Geometry check sheet. Reference: the model listing, model coordinates, mm. A direction names the side the tool comes from. Coordinates: 2 decimals unless noted, no trailing zeros. Write each loop counter-clockwise with the first axis right and the second up, starting at its lowest first coordinate (ties: lowest second). Pieces come first, ordered by that corner, then holes. Notation, with made-up numbers: (10, 63) -> (31, 63) arc R8 cw to (31, 76) -> close; hole circle Ø4 at (34.5, 80). An arc over 180 degrees is marked (long way). Use a Markdown table: item, result.
```python
from build123d import *

# Parameters (mm, degrees)
BOSS_EXTRUDE1_REACH     = 19.38
SKETCH3_W               = 4.76
SKETCH3_H               = 0.63
CUT_EXTRUDE1_DEPTH      = 19.196319901
CUT_EXTRUDE1_DEPTH_BACK = 19.196319901
SKETCH4_R               = 0.5


with BuildPart() as part:
    # Sweep1: sweep along a path in Sketch2
    with BuildLine(Plane(origin=(0, 0, 0), x_dir=(1, 0, 0), z_dir=(0, 1, 0))) as sweep1_path:
        Line((0, 2.62), (7, 2.62))
        Line((7, 2.62), (11.415258217, 3.755932179))
        ThreePointArc((11.415258217, 3.755932179), (13.415796262, 6.491493797), (11.121440392, 8.985763424))
        Line((11.121440392, 8.985763424), (6.606732095, 9.62))
        Line((6.606732095, 9.62), (0, 9.62))
        Line((0, 9.62), (0, 2.62))
    # Sketch1 → Sweep1 (sweep)
    with BuildSketch(Plane(origin=(0, 0, 0), x_dir=(0, 0, -1), z_dir=(1, 0, 0))):
        with BuildLine():
            Line((2.62, 0), (3.74, 0))
            Line((3.74, 0), (3.74, 0.63))
            Line((3.74, 0.63), (3.167964646, 0.63))
            ThreePointArc((3.167964646, 0.63), (2.881836518, 1.458738594), (2.383379953, 2.18))
            Line((2.383379953, 2.18), (1.496179773, 2.18))
            ThreePointArc((1.496179773, 2.18), (1.478667505, 2.178597055), (1.46160194, 2.174424008))
            ThreePointArc((1.46160194, 2.174424008), (2.312336165, 1.231869091), (2.62, 0))
        make_face()
    sweep(path=sweep1_path.line, transition=Transition.RIGHT)

    # Sketch3 → Boss-Extrude1 (add, up to next)
    with BuildSketch(Plane(origin=(1.12, 0, 0), x_dir=(0, 0, -1), z_dir=(1, 0, 0)), mode=Mode.PRIVATE) as boss_extrude1_sk1:
        with Locations((6.12, 0.315)):
            Rectangle(SKETCH3_W, SKETCH3_H)
    boss_extrude1_tool1 = extrude(boss_extrude1_sk1.sketch, amount=BOSS_EXTRUDE1_REACH, mode=Mode.PRIVATE) - part.part
    add(boss_extrude1_tool1.solids().sort_by_distance((1.12, 0.315, -6.12))[0])

    # Sketch4 → Cut-Extrude1 (cut, two sides: drawn at the far end of the back side and taken through both)
    with BuildSketch(Plane(origin=(0, 0.63, 0), x_dir=(1, 0, 0), z_dir=(0, 1, 0)).offset(-CUT_EXTRUDE1_DEPTH_BACK)):
        with Locations(Location((10.75, 6.341726352, 0), (0, 0, 270))):
            Circle(SKETCH4_R)
        with BuildLine():
            Line((1.497140147, 7.12), (1.497140147, 5.12))
            ThreePointArc((1.497140147, 5.12), (2.204246928, 4.827106781), (2.497140147, 4.12))
            Line((2.497140147, 4.12), (4.497140147, 4.12))
            ThreePointArc((4.497140147, 4.12), (4.790033365, 4.827106781), (5.497140147, 5.12))
            Line((5.497140147, 5.12), (5.497140147, 7.12))
            ThreePointArc((5.497140147, 7.12), (4.790033365, 7.412893219), (4.497140147, 8.12))
            Line((4.497140147, 8.12), (2.497140147, 8.12))
            ThreePointArc((2.497140147, 8.12), (2.204246928, 7.412893219), (1.497140147, 7.12))
        make_face()
    extrude(amount=CUT_EXTRUDE1_DEPTH + CUT_EXTRUDE1_DEPTH_BACK, mode=Mode.SUBTRACT)


solid = part.part
```
Item 1: Section check C-C on z = -6. Count the separate pieces of the cut face and the enclosed holes in it, then the cut area to 3 significant figures.
Answer block:
| item | result |
|---|---|
| separate pieces | 3 |
| enclosed holes | 0 |
| area | 7.74 mm^2 |
Item 2: Mould release check, pull along X, two halves, no side actions. Record for faces 1 (the cylindrical face through (2.21, 0.31, -7.42)), 2 (the cylindrical face through (9.243, 1.216, -2.888)), 3 (the cylindrical face through (3.05, 1.22, -2.32)): +X half, -X half, draft (parallel to the pull), parting line (faces both ways), or undercut.
Answer block:
| item | result |
|---|---|
| face 1 | undercut |
| face 2 | +X half |
| face 3 | draft |
Item 3: Section check B-B on y = 0.8. Record the boundary of the cut face in (x, z).
Answer block:
| item | result |
|---|---|
| outline | (-0.13, -9.75) -> (6.62, -9.75) -> (11.14, -9.11) arc R2.8 ccw to (11.45, -3.63) -> (7.02, -2.49) -> (-0.13, -2.49) -> close; hole (0.51, -9.11) -> (6.57, -9.11) -> (11.05, -8.48) arc R2.16 ccw to (11.29, -4.25) -> (6.94, -3.13) -> (0.51, -3.13) -> close |
Item 4: Depth check by flat-ended pin: P1, Ø0.7, axis at y = 0.5, z = -6.5, coming from the -X side; P2, Ø0.5, axis at x = 4, y = 0, coming from the -Z side; P3, Ø3, axis at x = 6, z = -7, coming from the +Y side. Enter the tip coordinate at first touch or a pass-through.
Answer block:
| item | result |
|---|---|
| P1 | stops at x = -0.14 |
| P2 | stops at z = -9.63 |
| P3 | stops at y = 0.63 |
Item 5: Thickness scan on L1, parallel to Y at x = 2, z = -3.75; L2, parallel to X at y = 2, z = -5.5; L3, parallel to Z at x = 10.75, y = 0.2. Record the ranges inside material, lowest first. Write a range as [from, to].
Answer block:
| item | result |
|---|---|
| L1 | y = [0, 0.63] |
| L2 | x = [-0.93, -0.08], [13.37, 14.25] |
| L3 | z = [-9.05, -6.84], [-5.84, -3.58] |
Item 6: Tool access check on faces 4 (the flat face through (7, 0.63, -6)), 5 (the cylindrical face through (2.2, 0.31, -4.83)), 6 (the flat face through (7, 0, -6)). Record the directions out of +Z, -Z, +X, -X, +Y, -Y that give a thin tool (end or side, any length) a straight path to the whole face; none if there is none.
Answer block:
| item | result |
|---|---|
| face 4 | +Y |
| face 5 | +Y, -Y |
| face 6 | +Z, -Z, +X, -X, -Y |
